```python
from build123d import *

# Parameters (mm, degrees)
EXTRUSION1_DEPTH      = 21
EXTRUSION1_DEPTH_BACK = 21
EXTRUSION2_DEPTH      = 14
SKIZZE3_R             = 8.05
EXTRUSION3_DEPTH      = 4.1
SKIZZE4_R             = 2.75
EXTRUSION4_DEPTH      = 4.1
SKIZZE5_R             = 2.75
EXTRUSION5_DEPTH      = 4.1


with BuildPart() as part:
    # Skizze1 → Extrusion1 (new body, two sides)
    with BuildSketch(Plane.XY) as extrusion1_sk:
        with BuildLine():
            Line((0, 40), (0, 5.6))
            ThreePointArc((0, 5.6), (1.640202025, 1.640202025), (5.6, 0))
            Line((5.6, 0), (20, 0))
            Line((20, 0), (20, 4))
            Line((20, 4), (5.6, 4))
            ThreePointArc((5.6, 4), (4.46862915, 4.46862915), (4, 5.6))
            Line((4, 5.6), (4, 40))
            Line((4, 40), (0, 40))
        make_face()
    extrude(amount=EXTRUSION1_DEPTH)
    extrude(extrusion1_sk.sketch, amount=-EXTRUSION1_DEPTH_BACK)

    # Skizze2 → Extrusion2 (cut, symmetric)
    with BuildSketch(Plane.YZ):
        with BuildLine():
            Line((64.1, 63.1), (-1, 63.1))
            Line((-1, 63.1), (-1, 23.320142873))
            Line((-1, 23.320142873), (25.188847397, 11.919557991))
            ThreePointArc((25.188847397, 11.919557991), (33, 0), (25.188847397, -11.919557991))
            Line((25.188847397, -11.919557991), (-1, -23.320142873))
            Line((-1, -23.320142873), (-1, -63.1))
            Line((-1, -63.1), (64.1, -63.1))
            Line((64.1, -63.1), (64.1, 63.1))
        make_face()
    extrude(amount=EXTRUSION2_DEPTH, both=True, mode=Mode.SUBTRACT)

    # Skizze3 → Extrusion3 (cut, symmetric)
    with BuildSketch(Plane.YZ):
        with Locations(Location((20, 0, 0), (0, 0, 90))):  # turned: the seam where the file's is
            Circle(SKIZZE3_R)
    extrude(amount=EXTRUSION3_DEPTH, both=True, mode=Mode.SUBTRACT)

    # Skizze4 → Extrusion4 (cut, symmetric)
    with BuildSketch(Plane(origin=(0, 0, 0), x_dir=(-1, 0, 0), z_dir=(0, 1, 0))):
        with Locations(Location((-14, -16, 0), (0, 0, 180))):  # turned: the seam where the file's is
            Circle(SKIZZE4_R)
    extrude(amount=EXTRUSION4_DEPTH, both=True, mode=Mode.SUBTRACT)

    # Skizze5 → Extrusion5 (cut, symmetric)
    with BuildSketch(Plane(origin=(0, 0, 0), x_dir=(-1, 0, 0), z_dir=(0, 1, 0))):
        with Locations(Location((-14, 16, 0), (0, 0, 180))):  # turned: the seam where the file's is
            Circle(SKIZZE5_R)
    extrude(amount=EXTRUSION5_DEPTH, both=True, mode=Mode.SUBTRACT)


solid = part.part
```
Input: part model. Units: mm. Frame: model coordinates. A direction names the side the tool comes from. Give positions to 0.01 mm unless a question says otherwise; leave off trailing zeros. Order: outer loops, then holes, each group sorted by start corner. A loop starts at its lowest first (then second) coordinate and runs counter-clockwise, first axis right, second up. Notation, with made-up numbers: (14, 16) -> (36, 16) arc R24 cw to (36, 54) -> close; hole circle Ø8 at (87.25, 18). An arc over 180 degrees is marked (long way). Write each question's results on one line, items separated by ' | '. Start each with the question number.
Item 1: Contact query for flat-ended pins moving along their axis: P1, Ø9, axis at x = 14, z = 16, coming from the +Y side; P2, Ø12, axis at y = 19, z = 9, coming from the +X side. Output: stop coordinate, or through.
Item 2: Cut plane C-C on x = 3. Return the cut outline in (y, z), then the cut area to 3 significant figures.
Item 3: Cut plane D-D on y = 20. Return the cut outline in (x, z), then the cut area to 3 significant figures.
Item 4: Line query: line 1 (Z direction, x = 14, y = 2.5); line 2 (Y direction, x = 14.5, z = -9); line 3 (Y direction, x = 2.45, z = 0). Output: solid intervals per line, ascending.
Item 5: Cut plane A-A on z = 0. Return the cut outline in (x, y), then the cut area to 3 significant figures.
Item 6: Cut plane B-B on x = 14. Return the cut outline in (y, z), then the cut area to 3 significant figures.
Item 7: Set-up query: faces 4 (the flat face through (10, 2, -21)), 5 (the flat face through (13, 4, 0)). Return all of +Z, -Z, +X, -X, +Y, -Y with unobstructed straight access to the full face (end or side cutting, diameter ignored); none if empty.
Item 8: Mould query, pull axis Z, two halves, no side actions, for faces 1 (the cylindrical face through (2.028, 27.859, -1.745)), 2 (the cylindrical face through (2, 33, 0)), 3 (the flat face through (4, 13, 5)). Classes: pulls with the +Z half, pulls with the -Z half, needs draft (parallel to the pull), parting line crosses it, or undercut.
Established:
1) P1: y = 4 | P2: x = 4
2) outline: (0.64, -21) -> (4.33, -21) -> (25.19, -11.92) arc R13 ccw to (25.19, 11.92) -> (4.33, 21) -> (0.64, 21) -> close; hole circle Ø16.1 at (20, 0) | area: 772 mm^2
3) outline: (0, -14.18) -> (4, -14.18) -> (4, -8.05) -> (0, -8.05) -> close; (0, 8.05) -> (4, 8.05) -> (4, 14.18) -> (0, 14.18) -> close | area: 49.0 mm^2
4) line 1: -21 to -18.75, -13.25 to 13.25, 18.75 to 21 | line 2: 0 to 4 | line 3: 0.97 to 11.95, 28.05 to 33
5) outline: (0, 5.6) arc R5.6 ccw to (5.6, 0) -> (20, 0) -> (20, 4) -> (5.6, 4) arc R1.6 cw to (4, 5.6) -> (4, 11.95) -> (0, 11.95) -> close; (0, 28.05) -> (4, 28.05) -> (4, 33) -> (0, 33) -> close | area: 125 mm^2
6) outline: (0, -21) -> (4, -21) -> (4, -18.75) -> (0, -18.75) -> close; (0, -13.25) -> (4, -13.25) -> (4, 13.25) -> (0, 13.25) -> close; (0, 18.75) -> (4, 18.75) -> (4, 21) -> (0, 21) -> close | area: 124 mm^2
7) face 4: -Z, +X, -X, +Y, -Y | face 5: +Z, -Z, +X, +Y
8) face 1: undercut | face 2: parting line crosses it | face 3: needs draft
